CAD build for the part. Positions are in the model's coordinates, mm. Round coordinates to 2 decimals unless told otherwise and drop trailing zeros. Loops run counter-clockwise (first coordinate to the right, second up) from the corner with the lowest first, then second, coordinate; pieces in that order, holes last.
from build123d import *

# Parameters (mm, degrees)
BOTTOM_R                    = 121
BOTTOM_R_2                  = 2.5
BOTTOM_W                    = 10
BOTTOM_H                    = 30
BOTTOM_EXTRUDE_DEPTH        = 4
HOLE_WIZARD_827_D           = 5.5
HOLE_WIZARD_827_DEPTH       = 20
HOLE_WIZARD_827_CSINK_D     = 10.4
HOLE_WIZARD_827_CSINK_ANGLE = 90
HOLE_WIZARD_827_TIP         = 1.652366702


with BuildPart() as part:
    # Bottom → Bottom-Extrude (new body)
    with BuildSketch(Plane(origin=(0, 0, 0), x_dir=(-1, 0, 0), z_dir=(0, 1, 0))):
        with Locations(Location((0, 0, 0), (0, 0, 90))):
            Circle(BOTTOM_R)
        with Locations(Location((-30.75, -24.25, 0), (0, 0, 90))):
            Circle(BOTTOM_R_2, mode=Mode.SUBTRACT)
        with Locations(Location((30.75, -24.25, 0), (0, 0, 90))):
            Circle(BOTTOM_R_2, mode=Mode.SUBTRACT)
        with Locations(Location((30.75, 24.25, 0), (0, 0, 90))):
            Circle(BOTTOM_R_2, mode=Mode.SUBTRACT)
        with Locations(Location((-30.75, 24.25, 0), (0, 0, 90))):
            Circle(BOTTOM_R_2, mode=Mode.SUBTRACT)
        with Locations((100, 0)):
            Rectangle(BOTTOM_W, BOTTOM_H, mode=Mode.SUBTRACT)
        with Locations((-100, 0)):
            Rectangle(BOTTOM_W, BOTTOM_H, mode=Mode.SUBTRACT)
    extrude(amount=BOTTOM_EXTRUDE_DEPTH)

    # Hole Wizard 827
    with Locations(Plane(origin=(-40.138590538, 0, -6.235728401), x_dir=(0.8690947690911651, 0, 0.49464561287691045), z_dir=(0, -1, 0))):
        with Locations((-45.469885408, -97.873538962), (-80.031285228, -14.434938782), (-45.469885408, 69.003661398), (37.968714772, 103.565061218), (121.407314952, 69.003661398), (155.968714772, -14.434938782), (121.407314952, -97.873538962), (37.968714772, -132.434938782)):
            CounterSinkHole(HOLE_WIZARD_827_D / 2, HOLE_WIZARD_827_CSINK_D / 2, depth=HOLE_WIZARD_827_DEPTH, counter_sink_angle=HOLE_WIZARD_827_CSINK_ANGLE)
            with Locations((0, 0, -(HOLE_WIZARD_827_DEPTH + HOLE_WIZARD_827_TIP / 2))):  # 118° drill point
                Cone(0, HOLE_WIZARD_827_D / 2, HOLE_WIZARD_827_TIP, mode=Mode.SUBTRACT)


solid = part.part
Item 1: Cut at A-A (z = 0). List the corners of the cut face in (x, y), plus the area to 3 significant figures.
Verdict:
outline: (-121, 0) - (-105, 0) - (-105, 4) - (-121, 4) - close; (-95, 0) - (95, 0) - (95, 4) - (-95, 4) - close; (105, 0) - (121, 0) - (121, 4) - (105, 4) - close
area: 888 mm2
Item 2: Flat gauge pins, fed straight in: P1, Ø1.2, axis at y = 3, z = 7.5, coming from the -X side; P2, Ø1, axis at y = 1, z = -60, coming from the +X side; P3, Ø1.2, axis at x = 102.5, y = 2.5, coming from the -Z side. Where does each tip first touch, or does it go through?
Verdict:
P1: stops at x = -120.8
P2: stops at x = 105.36
P3: stops at z = -65.25
Item 3: Mould opens along Z. For faces 1 (the cylindrical face through (-118.123, 1.972, -26.23)), 2 (the cylindrical face through (-60.055, 3.236, 100.381)), 3 (the cylindrical face through (-111.064, 3.236, 30.869)), 4 (the flat face through (2, 4, -2)) say: released by +Z, released by -Z, zero draft, split by the parting line, or undercut.
Verdict:
face 1: split by the parting line
face 2: undercut
face 3: undercut
face 4: zero draft
Item 4: Cut at D-D (z = 71.5). List the corners of the cut face in (x, y).
Verdict:
outline: (-97.62, 0) - (97.62, 0) - (97.62, 4) - (-97.62, 4) - close
Item 5: Wall check: L1, parallel to X at y = 3.2, z = -11.5; L2, parallel to X at y = 1.8, z = -24.5; L3, parallel to Z at x = -96, y = 1.35. Give the ranges that are in metal, low to high.
Verdict:
L1: x = -120.45 to -105, -95 to 95, 105 to 120.45
L2: x = -118.49 to -33.24, -28.26 to 28.26, 33.24 to 118.49
L3: z = -73.65 to -15, 15 to 73.65
Item 6: Cut at C-C (x = 72.5). List the corners of the cut face in (y, z), plus the area to 3 significant figures.
Verdict:
outline: (0, -96.87) - (4, -96.87) - (4, 96.87) - (0, 96.87) - close
area: 775 mm2
Item 7: Cut at B-B (y = 3.2). State how many separate pieces and enclosed holes the cut face has, plus the area to 3 significant figures.
Verdict:
separate pieces: 1
enclosed holes: 14
area: 45,100 mm2
